Read the model definition and answer for the solid it produces. Units are mm, in the model's axes. Give positions to 0.01 mm unless a question says otherwise; leave off trailing zeros. Order: outer loops, then holes, each group sorted by start corner. A loop starts at its lowest first (then second) coordinate and runs counter-clockwise, first axis right, second up. Notation, with made-up numbers: (-32.75, 44) - (-14.75, 44) arc R23 cw to (-14.75, 66) - close; hole circle Ø5 at (58.25, 17). An arc over 180 degrees is marked (long way). Return JSON: item names as keys, results as strings.
```python
from build123d import *

# Parameters (mm, degrees)
F1_DEPTH = 1.3
F2_DEPTH = 17
F4_DEPTH = 5


# Not quite as in the source:
# - a feature names something its author has since deleted; it is built from what else it names


with BuildPart() as f1:
    # F0 (on Top) → F1 (new body)
    with BuildSketch(Plane.XY):
        Polygon((24, 57.25), (-24, 57.25), (-24.0091441598, 54.25), (-22.5091511277, 54.2454279414), (-22.5091511277, 42.2454279414), (-22.4957785658, -34.7500035641), (-22.5, -49.25), (-24, -49.25), (-24, -57.25), (24, -57.25), align=None)
        with BuildLine():
            Line((13.9209458456, -22.2416133583), (-17.6390541544, -22.2416133583))
            ThreePointArc((-17.6390541544, -22.2416133583), (-19.8890541544, -19.9916133583), (-17.6390541544, -17.7416133583))
            Line((-17.6390541544, -17.7416133583), (13.9209458456, -17.7416133583))
            ThreePointArc((13.9209458456, -17.7416133583), (16.1709458456, -19.9916133583), (13.9209458456, -22.2416133583))
        make_face(mode=Mode.SUBTRACT)
        with BuildLine():
            Line((9.9809458456, -13.7416133583), (-17.6390541544, -13.7416133583))
            ThreePointArc((-17.6390541544, -13.7416133583), (-19.8890541544, -11.4916133583), (-17.6390541544, -9.2416133583))
            Line((-17.6390541544, -9.2416133583), (9.9809458456, -9.2416133583))
            ThreePointArc((9.9809458456, -9.2416133583), (12.2309458456, -11.4916133583), (9.9809458456, -13.7416133583))
        make_face(mode=Mode.SUBTRACT)
        with BuildLine():
            Line((6.0409458456, -5.2416133583), (-17.6390541544, -5.2416133583))
            ThreePointArc((-17.6390541544, -5.2416133583), (-19.8890541544, -2.9916133583), (-17.6390541544, -0.7416133583))
            Line((-17.6390541544, -0.7416133583), (6.0409458456, -0.7416133583))
            ThreePointArc((6.0409458456, -0.7416133583), (8.2909458456, -2.9916133583), (6.0409458456, -5.2416133583))
        make_face(mode=Mode.SUBTRACT)
        with BuildLine():
            Line((-19.9999999992, -31.5317022603), (-19.9999999992, -27.0317022603))
            Line((-19.9999999992, -27.0317022603), (16.0951670268, -27.0317022603))
            ThreePointArc((16.0951670268, -27.0317022603), (18.3824934665, -27.555243649), (19.9999999704, -29.25513498))
            Line((19.9999999704, -29.25513498), (19.991580365, -37.75513498))
            Line((19.991580365, -37.75513498), (6.1573753969, -37.7551350426))
            ThreePointArc((6.1573753969, -37.7551350426), (5.4441089744, -38.037790108), (4.9890264818, -38.6554816172))
            Line((4.9890264818, -38.6554816172), (4.9890264818, -40.6197120801))
            Line((4.9890264818, -40.6197120801), (19.9890264818, -40.6197120801))
            Line((19.9890264818, -40.6197120801), (20, -44.6197120801))
            Line((20, -44.6197120801), (0, -44.6197120801))
            Line((0, -44.6197120801), (0, -37.7900532508))
            ThreePointArc((0, -37.7900532508), (1.5958871284, -35.3350022858), (4.3312619815, -34.2900834468))
            Line((4.3312619815, -34.2900834468), (14.5000001306, -34.2900834468))
            Line((14.5000001306, -34.2900834468), (14.5000000048, -32.3122422563))
            ThreePointArc((14.5000000048, -32.3122422563), (14.2713851276, -31.7603171319), (13.7194600008, -31.5317022603))
            Line((13.7194600008, -31.5317022603), (-7.2499999992, -31.5317022603))
            Line((-7.2499999992, -31.5317022603), (-7.2499999992, -44.8960133593))
            Line((-7.2499999992, -44.8960133593), (-12.7499999992, -44.8960133593))
            Line((-12.7499999992, -44.8960133593), (-12.7499999992, -31.5317022603))
            Line((-12.7499999992, -31.5317022603), (-19.9999999992, -31.5317022603))
        make_face(mode=Mode.SUBTRACT)
        with BuildLine():
            Line((2.1009458456, 3.2583866417), (-17.6390541544, 3.2583866417))
            ThreePointArc((-17.6390541544, 3.2583866417), (-19.8890541544, 5.5083866417), (-17.6390541544, 7.7583866417))
            Line((-17.6390541544, 7.7583866417), (2.1009458456, 7.7583866417))
            ThreePointArc((2.1009458456, 7.7583866417), (4.3509458456, 5.5083866417), (2.1009458456, 3.2583866417))
        make_face(mode=Mode.SUBTRACT)
        with BuildLine():
            Line((-2.5590541544, 11.7583866417), (-17.6390541544, 11.7583866417))
            ThreePointArc((-17.6390541544, 11.7583866417), (-19.8890541544, 14.0083866417), (-17.6390541544, 16.2583866417))
            Line((-17.6390541544, 16.2583866417), (-2.5590541544, 16.2583866417))
            ThreePointArc((-2.5590541544, 16.2583866417), (-0.3090541544, 14.0083866417), (-2.5590541544, 11.7583866417))
        make_face(mode=Mode.SUBTRACT)
        with BuildLine():
            Line((-5.7790541544, 20.2583866417), (-17.6390541544, 20.2583866417))
            ThreePointArc((-17.6390541544, 20.2583866417), (-19.8890541544, 22.5083866417), (-17.6390541544, 24.7583866417))
            Line((-17.6390541544, 24.7583866417), (-5.7790541544, 24.7583866417))
            ThreePointArc((-5.7790541544, 24.7583866417), (-3.5290541544, 22.5083866417), (-5.7790541544, 20.2583866417))
        make_face(mode=Mode.SUBTRACT)
        with BuildLine():
            Line((-9.7190541544, 28.7583866417), (-17.6390541544, 28.7583866417))
            ThreePointArc((-17.6390541544, 28.7583866417), (-19.8890541544, 31.0083866417), (-17.6390541544, 33.2583866417))
            Line((-17.6390541544, 33.2583866417), (-9.7190541544, 33.2583866417))
            ThreePointArc((-9.7190541544, 33.2583866417), (-7.4690541544, 31.0083866417), (-9.7190541544, 28.7583866417))
        make_face(mode=Mode.SUBTRACT)
        with BuildLine():
            Line((-13.6590541544, 37.2583866417), (-17.6390541544, 37.2583866417))
            ThreePointArc((-17.6390541544, 37.2583866417), (-19.8890541544, 39.5083866417), (-17.6390541544, 41.7583866417))
            Line((-17.6390541544, 41.7583866417), (-13.6590541544, 41.7583866417))
            ThreePointArc((-13.6590541544, 41.7583866417), (-11.4090541544, 39.5083866417), (-13.6590541544, 37.2583866417))
        make_face(mode=Mode.SUBTRACT)
        with BuildLine():
            Line((-17.5990541544, 45.7583866417), (-17.6390541544, 45.7583866417))
            ThreePointArc((-17.6390541544, 45.7583866417), (-19.8890541544, 48.0083866417), (-17.6390541544, 50.2583866417))
            Line((-17.6390541544, 50.2583866417), (-17.5990541544, 50.2583866417))
            ThreePointArc((-17.5990541544, 50.2583866417), (-15.3490541544, 48.0083866417), (-17.5990541544, 45.7583866417))
        make_face(mode=Mode.SUBTRACT)
    extrude(amount=-F1_DEPTH)

    # F0 (on Top) → F2 (join)
    with BuildSketch(Plane.XY):
        Polygon((-22.5091511277, 54.2454279414), (-24.0091441598, 54.25), (-23.9065294749, 42.2334950591), (-22.5091511277, 42.2454279414), align=None)
        Polygon((-22.4957785658, -34.7500035641), (-23.9957785658, -34.7500035641), (-24, -49.25), (-22.5, -49.25), align=None)
    extrude(amount=-F2_DEPTH)

    # F0 (on Top) → F4 (join)
    with BuildSketch(Plane.XY):
        Polygon((-22.5091511277, 42.2454279414), (-23.9065294749, 42.2334950591), (-23.9957785658, -34.7500035641), (-22.4957785658, -34.7500035641), align=None)
    extrude(amount=-F4_DEPTH)


solid = f1.part
```
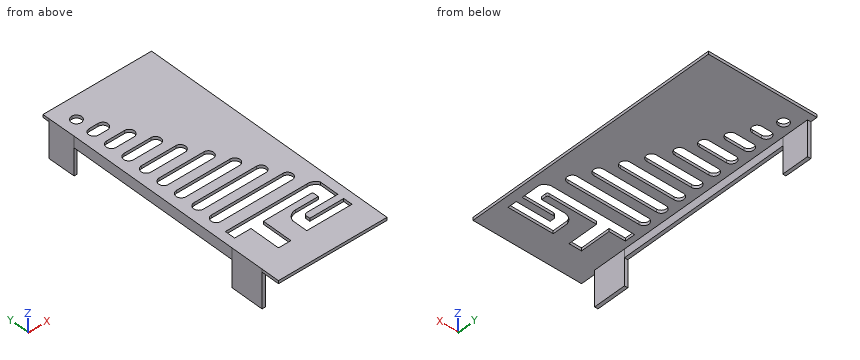
Q1. A cutting plane is placed at A-A (z = -10). Write down the section's boundary in (x, y), and give its area (3 significant figures).
Values:
{"outline": "(-24.01, 54.25) - (-23.91, 42.23) - (-22.51, 42.25) - (-22.51, 54.25) - close; (-24, -49.25) - (-22.5, -49.25) - (-22.5, -34.75) - (-24, -34.75) - close", "area": "39.1 mm²"}
Q2. A cutting plane is placed at B-B (y = -36). Write down the section's boundary in (x, z), and give its area (3 significant figures).
Values:
{"outline": "(-24, -17) - (-22.5, -17) - (-22.5, -1.3) - (-12.75, -1.3) - (-12.75, 0) - (-24, 0) - close; (-7.25, -1.3) - (0.92, -1.3) - (0.92, 0) - (-7.25, 0) - close; (19.99, -1.3) - (24, -1.3) - (24, 0) - (19.99, 0) - close", "area": "54.0 mm²"}
Q3. Consider L1, parallel to X at y = 44.5, z = -5.5; L2, parallel to Z at x = 10, y = -25.5; L3, parallel to X at y = -29, z = -2.5. Determine where each line is inside the solid, lowest interval first.
Values:
{"L1": "x = -23.93 to -22.51", "L2": "z = -1.3 to 0", "L3": "x = -23.99 to -22.5"}
Q4. A cutting plane is placed at C-C (z = -3). Write down the section's boundary in (x, y).
Values:
{"outline": "(-24.01, 54.25) - (-23.91, 42.23) - (-24, -34.75) - (-24, -49.25) - (-22.5, -49.25) - (-22.5, -34.75) - (-22.51, 42.25) - (-22.51, 54.25) - close"}
Q5. Given pin 1 (0.8 mm diameter, centred on x = -23, z = -12.5, fed in from -Y); pin 2 (1.2 mm diameter, centred on x = -23, y = -8.5, fed in from -Z); pin 3 (10 mm diameter, centred on x = -5, y = 2, fed in from -Z), each flat-ended and moving along its own axis, determine where each tip first touches the part or whether it passes through.
Values:
{"pin 1": "stops at y = -49.25", "pin 2": "stops at z = -5", "pin 3": "stops at z = -1.3"}
